CAD build for the part. Positions are in the model's coordinates, mm. Face numbers are marked on the shaded views. A direction names the side the tool comes from. Coordinates: 2 decimals unless noted, no trailing zeros. Order: outer loops, then holes, each group sorted by start corner. A loop starts at its lowest first (then second) coordinate and runs counter-clockwise, first axis right, second up. Notation, with made-up numbers: (-34.75, 74) - (1.25, 74) arc R13 ccw to (1.25, 86) - close; hole circle Ø5 at (38, -34). An arc over 180 degrees is marked (long way). Use one line per item in the form item = value.
```python
from build123d import *

# Parameters (mm, degrees)
F1_DEPTH  = 12.7
F3_R      = 31.75
F3_R_2    = 22.225
F4_DEPTH  = 12.7
F5_R      = 1.5875
F5_R_2    = 3.175
F6_DEPTH  = 203.2
F10_DEPTH = 304.8
F11_W     = 349.25
F11_H     = 152.4
F12_DEPTH = 876.3010001


# Not quite as in the source:
# - ends of sketch curves that miss each other by under 0.0002 mm in the source are joined
# - a feature of the source that left no trace in its solid (it failed there, or was rolled back) is left out
# - a pattern or mirror of a feature is missing from the dataset's text; its kind, count and spacing are read off the source's solid


with BuildPart() as f1:
    # F0 (on Top) → F1 (new body)
    with BuildSketch(Plane.XY):
        with BuildLine():
            Line((-599.0488908, 46.9398096), (-599.0488908, 40.5898096))
            ThreePointArc((-599.0488908, 40.5898096), (-597.1890188605, 36.0996815395), (-592.6988908, 34.2398096))
            Line((-592.6988908, 34.2398096), (-522.8488908, 34.2398096))
            add(Edge.make_bspline(
                [(-268.8488908, -83.2351904), (-268.8488908, 34.2397712098), (-522.8488908, 34.2398096)],
                knots=[0, 0, 0, 1.570796, 1.570796, 1.570796], degree=2, weights=[1, 0.7071068967, 1]))
            Line((-268.8488908, -83.2351904), (-268.8488908, -438.8351904))
            ThreePointArc((-268.8488908, -438.8351904), (-265.1291469211, -447.8154465211), (-256.1488908, -451.5351904))
            Line((-256.1488908, -451.5351904), (448.7011092, -451.5351904))
            ThreePointArc((448.7011092, -451.5351904), (457.6813653211, -447.8154465211), (461.4011092, -438.8351904))
            Line((461.4011092, -438.8351904), (461.4011092, -83.2351904))
            add(Edge.make_bspline(
                [(715.4011042177, 34.2398096), (461.4011872236, 34.2398072957), (461.4011092, -83.2351904)],
                knots=[4.712389, 4.712389, 4.712389, 6.283185, 6.283185, 6.283185], degree=2, weights=[1, 0.7071068967, 1]))
            Line((715.4011042177, 34.2398096), (785.2511092, 34.2398096))
            ThreePointArc((785.2511092, 34.2398096), (789.7412372605, 36.0996815395), (791.6011092, 40.5898096))
            Line((791.6011092, 40.5898096), (791.6011092, 46.9398096))
            ThreePointArc((791.6011092, 46.9398096), (753.9970119259, 191.9633164225), (650.6608007323, 300.4414852816))
            ThreePointArc((650.6608007323, 300.4414852816), (535.0314824748, 358.4359268507), (410.8101236244, 394.5267587894))
            ThreePointArc((410.8101236244, 394.5267587894), (96.2761092, 424.7648096), (-218.2579085609, 394.5267759822))
            ThreePointArc((-218.2579085609, 394.5267759822), (-342.4792640748, 358.4359268507), (-458.1085745053, 300.4414726845))
            ThreePointArc((-458.1085745053, 300.4414726845), (-561.4447935259, 191.9633164225), (-599.0488908, 46.9398096))
        make_face()
    extrude(amount=F1_DEPTH)

    # F3 (on offset) → F4 (join)
    with BuildSketch(Plane.YZ.offset(279.4)):
        with Locations((-420.6445217133, 41.4921417832)):
            Circle(F3_R)
        with Locations((-420.6445217133, 41.4921417832)):
            Circle(F3_R_2, mode=Mode.SUBTRACT)
    f4 = extrude(amount=F4_DEPTH)

    # F4_copies: F4 across plane
    add(f4.mirror(Plane(origin=(96.276109, 0, 0), x_dir=(0, 0, -1), z_dir=(-1, 0, 0))))

    # F5 (on face) → F6 (join)
    with BuildSketch(Plane.XY.offset(12.7)):
        with Locations((545.5359220505, 190.6074881554)):
            Circle(F5_R)
        with Locations((280.7082656561, 252.0138544033)):
            Circle(F5_R_2)
    f6 = extrude(amount=F6_DEPTH)

    # F6_copies: F6 across plane
    add(f6.mirror(Plane(origin=(96.276109, 0, 0), x_dir=(0, 0, -1), z_dir=(-1, 0, 0))))

    # F9 (on face) → F10 (join)
    with BuildSketch(Plane.XY.offset(12.7)):
        with BuildLine():
            Line((734.4511103495, 46.9398096), (740.8011092, 46.9398096))
            ThreePointArc((740.8011092, 46.9398096), (709.5977093343, 167.2784641974), (623.8506404715, 257.292263889))
            ThreePointArc((623.8506404715, 257.292263889), (516.4805587409, 311.1442444042), (401.1321540941, 344.6571597759))
            ThreePointArc((401.1321540941, 344.6571597759), (96.2761092, 373.9648096), (-208.5799387837, 344.6571770166))
            ThreePointArc((-208.5799387837, 344.6571770166), (-323.9283403409, 311.1442444042), (-431.2984143121, 257.2922512499))
            ThreePointArc((-431.2984143121, 257.2922512499), (-517.0454909343, 167.2784641974), (-548.2488908, 46.9398096))
            Line((-548.2488908, 46.9398096), (-541.8989002521, 46.9398096))
            ThreePointArc((-541.8989002521, 46.9398096), (-511.4955863715, 164.1928622622), (-427.9471570273, 251.8986192435))
            ThreePointArc((-427.9471570273, 251.8986192435), (-321.6094769175, 305.2327893075), (-207.3701905688, 338.4234653923))
            ThreePointArc((-207.3701905688, 338.4234653923), (96.2761092, 367.6148096), (399.9224109615, 338.4234771459))
            ThreePointArc((399.9224109615, 338.4234771459), (514.1616980249, 305.2327962096), (620.4993695539, 251.8986096209))
            ThreePointArc((620.4993695539, 251.8986096209), (704.047797515, 164.1928582278), (734.4511103495, 46.9398096))
        make_face()
    extrude(amount=F10_DEPTH)

    # F11 (on face) → F12 (cut, through all)
    with BuildSketch(Plane.XZ.offset(451.5351904)):
        with Locations((96.2761092, 88.9)):
            Rectangle(F11_W, F11_H)
    extrude(amount=-F12_DEPTH, mode=Mode.SUBTRACT)


solid = f1.part
```
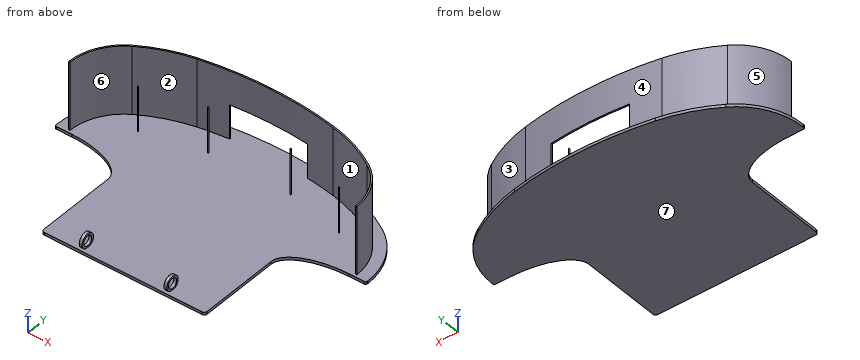
Item 1: Cut at B-B, the plane x = 237. Write the cut outline in (y, z), plus the area to 3 significant figures.
Derived:
outline = (-451.54, 0) - (418.76, 0) - (418.76, 12.7) - (-451.54, 12.7) - close; (361.39, 165.1) - (367.77, 165.1) - (367.77, 317.5) - (361.39, 317.5) - close
area = 12,000 mm²
Item 2: Cut at D-D, the plane y = 161. Write the cut outline in (x, z).
Derived:
outline = (-576.39, 0) - (768.95, 0) - (768.95, 12.7) - (712.97, 12.7) - (712.97, 317.5) - (705.79, 317.5) - (705.79, 12.7) - (-513.24, 12.7) - (-513.24, 317.5) - (-520.42, 317.5) - (-520.42, 12.7) - (-576.39, 12.7) - close
Item 3: Two-plate mould, pull along X, no slides. Class the marked faces 1, 2, 3 and 4: +X half, -X half, draft (parallel to the pull), parting line (faces both ways), or undercut.
Derived:
face_1 = undercut
face_2 = undercut
face_3 = +X half
face_4 = parting line
Item 4: Drill centre lines: line 1 (Z direction, x = 102.5, y = 173); line 2 (X direction, y = 226, z = 189); line 3 (X direction, y = 206.5, z = 136). Where is each one in solid material? Low to high. Write a range as [from, to].
Derived:
line_1 = [0, 12.7]
line_2 = [-471.68, -462.35], [654.9, 664.23]
line_3 = [-490, -481.61], [674.17, 682.55]
Item 5: Cut at A-A, the plane z = 252. Write the cut outline in (x, y).
Derived:
outline = (-548.25, 46.94) - (-541.9, 46.94) arc R241.3 cw to (-427.95, 251.9) arc R654.05 cw to (-207.37, 338.42) arc R1593.85 cw to (399.92, 338.42) arc R654.05 cw to (620.5, 251.9) arc R241.3 cw to (734.45, 46.94) - (740.8, 46.94) arc R247.65 ccw to (623.85, 257.29) arc R660.4 ccw to (401.13, 344.66) arc R1600.2 ccw to (-208.58, 344.66) arc R660.4 ccw to (-431.3, 257.29) arc R247.65 ccw to start
Item 6: 3-axis set-ups, long thin cutter, end or side, ignore diameter. For the marked faces 5, 6 and 7: which of +Z, -Z, +X, -X, +Y, -Y reach the whole face in a straight line?
Derived:
face_5 = +Z, -X, +Y
face_6 = +Z, -Y
face_7 = -Z, +X, -X, +Y, -Y
Item 7: Cut at C-C, the plane z = 126. State how many separate pieces and enclosed holes the cut face has, plus the area to 3 significant figures.
Derived:
separate_pieces = 6
enclosed_holes = 0
area = 7,940 mm²
Item 8: Drop flat-ended pins along their axis: pin 1 (4 mm diameter, centred on x = 750, z = 8, fed in from -Y); pin 2 (6 mm diameter, centred on y = 125.5, z = 249.5, fed in from -X); pin 3 (10 mm diameter, centred on y = -343.5, z = 7, fed in from +X). Give the stop position or say it passes through.
Derived:
pin_1 = 34.24
pin_2 = -536.44
pin_3 = 461.4
